from build123d import *

# Parameters (mm, degrees)
BOSS_EXTRU_1_DEPTH           = 15
ENL_V_START                  = 7.5
ESQUISSE2_R                  = 10
ENL_V_MAT_EXTRU_1_DEPTH      = 6.25
R_P_TITION_CIRCULAIRE1_COUNT = 3
TROU_TARAUD_M81_D            = 6.8
TROU_TARAUD_M81_CSINK_D      = 8.05
TROU_TARAUD_M81_CSINK_ANGLE  = 90
ESQUISSE7_R                  = 7.460158596
ESQUISSE7_R_2                = 5.383247208
BOSS_EXTRU_2_DEPTH           = 12.5
ESQUISSE7_3_R                = 5.383247208
ENL_V_MAT_EXTRU_2_DEPTH      = 66.766038545


with BuildPart() as part:
    # Esquisse1 → Boss.-Extru.1 (new body)
    with BuildSketch(Plane.XY):
        with BuildLine():
            Line((-8.660254038, 42.735026919), (-41.339745962, -13.867513459))
            ThreePointArc((-41.339745962, -13.867513459), (-41.339745962, -23.867513459), (-32.679491924, -28.867513459))
            Line((-32.679491924, -28.867513459), (32.679491924, -28.867513459))
            ThreePointArc((32.679491924, -28.867513459), (41.339745962, -23.867513459), (41.339745962, -13.867513459))
            Line((41.339745962, -13.867513459), (8.660254038, 42.735026919))
            ThreePointArc((8.660254038, 42.735026919), (0, 47.735026919), (-8.660254038, 42.735026919))
        make_face()
    extrude(amount=BOSS_EXTRU_1_DEPTH)

    # Esquisse2 → Enl_v. mat.-Extru.1 (cut, symmetric)
    with BuildSketch(Plane.XY.offset(ENL_V_START)):
        with Locations((0, 37.735026919)):
            Circle(ESQUISSE2_R)
    enl_v_mat_extru_1 = extrude(amount=ENL_V_MAT_EXTRU_1_DEPTH, both=True, mode=Mode.SUBTRACT)

    # R_p_tition circulaire1: Enl_v. mat.-Extru.1 ×3 about axis
    r_p_tition_circulaire1_axis = Axis((0, 0, 0), (0, 0, 1))
    for i in range(1, R_P_TITION_CIRCULAIRE1_COUNT):
        add(enl_v_mat_extru_1.rotate(r_p_tition_circulaire1_axis, i * 360 / R_P_TITION_CIRCULAIRE1_COUNT), mode=Mode.SUBTRACT)

    # Trou taraud_ M81 (through all)
    with Locations(Plane(origin=(0, 0, 0), x_dir=(-1, 0, 0), z_dir=(0, 0, -1))):
        with Locations((0, 37.735026919), (32.679491924, -18.867513459), (-32.679491924, -18.867513459)):
            CounterSinkHole(TROU_TARAUD_M81_D / 2, TROU_TARAUD_M81_CSINK_D / 2, counter_sink_angle=TROU_TARAUD_M81_CSINK_ANGLE)

    # Esquisse7 → Boss.-Extru.2 (add)
    with BuildSketch(Plane(origin=(0, 0, 0), x_dir=(-1, 0, 0), z_dir=(0, 0, -1))):
        with Locations(Location((0, 0, 0), (0, 0, 180))):
            Circle(ESQUISSE7_R)
        Circle(ESQUISSE7_R_2, mode=Mode.SUBTRACT)
    extrude(amount=BOSS_EXTRU_2_DEPTH)

    # Esquisse7_3 → Enl_v. mat.-Extru.2 (cut, through all)
    with BuildSketch(Plane(origin=(0, 0, 0), x_dir=(-1, 0, 0), z_dir=(0, 0, -1))):
        Circle(ESQUISSE7_3_R)
    extrude(amount=-ENL_V_MAT_EXTRU_2_DEPTH, mode=Mode.SUBTRACT)


solid = part.part
Input: part model. Units: mm. Frame: model coordinates. A direction names the side the tool comes from. Give positions to 0.01 mm unless a question says otherwise; leave off trailing zeros. Order: outer loops, then holes, each group sorted by start corner. A loop starts at its lowest first (then second) coordinate and runs counter-clockwise, first axis right, second up. Notation, with made-up numbers: (65, 83.5) - (116, 83.5) arc R6 cw to (116, 91.5) - close; hole circle Ø2 at (3.5, 30.25). An arc over 180 degrees is marked (long way). Answer as a JSON object with one key per item and string values. Group by question number.
Q1. Cut plane B-B, the plane y = -1. Output: boundary loops of the cut face in (x, z), then the cut area to 3 significant figures.
Q2. Set-up query: faces 5 (the face through (4, -4, -12.5)), 6 (the face through (-0.29, 27.74, 7.59)). Return all of +Z, -Z, +X, -X, +Y, -Y with unobstructed straight access to the full face (end or side cutting, diameter ignored); none if empty.
Q3. Cut plane C-C, the plane z = 4.5. Output: boundary loops of the cut face in (x, y).
Q4. First-contact query: pin 1 Ø16 at (x, y) = (-32.68, -18.87) entering from -Z; pin 2 Ø10 at (x, z) = (-22, 12) entering from +Y. Flat tips, straight axial feed; report the tip coordinate or a pass-through.
Q5. Mould query, pull axis Z, two halves, no side actions, for faces 1 (the face through (-0.443, 41.106, 14.384)), 2 (the face through (31, -23, 13.75)), 3 (the face through (9, 1, 0)), 4 (the face through (-29, -17, 1.25)). Classes: pulls with the +Z half, pulls with the -Z half, needs draft (parallel to the pull), parting line crosses it, or undercut.
Q6. Line query: probe 1 along Y at (x, z) = (0, 0.85); probe 2 along Z at (x, y) = (-8, 40.5); probe 3 along Y at (x, z) = (0, 6.5). Output: solid intervals per line, ascending.
Q7. Cut plane A-A, the plane x = 0. Output: boundary loops of the cut face in (y, z) (3 decimals), then the cut area to 3 significant figures.
Q8. Cut plane D-D, the plane y = 30. Output: boundary loops of the cut face in (x, z).
Results:
{
 "1": {"outline": "(-33.91, 0) - (-7.39, 0) - (-7.39, -12.5) - (-5.29, -12.5) - (-5.29, 15) - (-33.91, 15) - close; (5.29, -12.5) - (7.39, -12.5) - (7.39, 0) - (33.91, 0) - (33.91, 15) - (5.29, 15) - close", "area": "911 mm^2"},
 "2": {"face 5": "-Z, +X, -X, +Y, -Y", "face 6": "none"},
 "3": {"outline": "(-41.34, -13.87) arc R10 cw (long way) to (-32.68, -28.87) - (32.68, -28.87) arc R10 cw (long way) to (41.34, -13.87) - (8.66, 42.74) arc R10 cw (long way) to (-8.66, 42.74) - close; hole circle Ø10.77 at (0, 0)"},
 "4": {"pin 1": "z = 0", "pin 2": "y = 28.29"},
 "5": {"face 1": "needs draft", "face 2": "undercut", "face 3": "pulls with the -Z half", "face 4": "undercut"},
 "6": {"probe 1": "-28.87 to -5.38, 5.38 to 34.34, 41.14 to 47.74", "probe 2": "0 to 1.25, 13.75 to 15", "probe 3": "-28.87 to -5.38, 5.38 to 27.74"},
 "7": {"outline": "(-28.868, 0) - (-7.46, 0) - (-7.46, -12.5) - (-5.383, -12.5) - (-5.383, 15) - (-28.868, 15) - close; (5.383, -12.5) - (7.46, -12.5) - (7.46, 0) - (33.71, 0) - (34.335, 0.625) - (34.335, 1.25) - (27.735, 1.25) - (27.735, 13.75) - (34.335, 13.75) - (34.335, 15) - (5.383, 15) - close; (41.135, 0.625) - (41.76, 0) - (47.735, 0) - (47.735, 1.25) - (41.135, 1.25) - close; (41.135, 13.75) - (47.735, 13.75) - (47.735, 15) - (41.135, 15) - close", "area": "772 mm^2"},
 "8": {"outline": "(-16.01, 0) - (16.01, 0) - (16.01, 15) - (-16.01, 15) - close; hole (-6.34, 1.25) - (6.34, 1.25) - (6.34, 13.75) - (-6.34, 13.75) - close"}
}
